Input: part model. Units: mm. Frame: model coordinates. A direction names the side the tool comes from. Coordinates: 2 decimals unless noted, no trailing zeros. Loops run counter-clockwise (first coordinate to the right, second up) from the corner with the lowest first, then second, coordinate; pieces in that order, holes last. Notation, with made-up numbers: M 27.25,50 L 59.25,50 A16 ccw 59.25,76 Z; hole C 69,-11 d11. An arc over 180 degrees is marked long. Use a Markdown table: item, result. Add a question column.
1. Section C-C on y = -2.5. Output: boundary loops of the cut face in (x, z).
2. Section D-D on z = 0. Output: boundary loops of the cut face in (x, y), then the cut area to 3 significant figures.
3. Draft query along X for faces 4 (the flat face through (-5, -0.5, -0.1)), 5 (the flat face through (0, -1, -6)), 6 (the flat face through (0, -4, 10)), 7 (the flat face through (-15.5, -8.5, 0)). Return one class per face: +X half, -X half, draft (parallel to the pull), parting line (faces both ways), or undercut.
4. Section A-A on z = -3. Output: boundary loops of the cut face in (x, y).
5. Pin query (flat end, axial travel): pin 1 (0.5 mm diameter, centred on y = -0.5, z = 1, fed in from +X); pin 2 (1.1 mm diameter, centred on x = 12, y = -8.5, fed in from -Z); pin 3 (2.5 mm diameter, centred on x = 13, z = 0.5, fed in from +Y). Return the tip coordinate at first contact, or that it passes through.
6. Line query: L1, parallel to Z at x = 3.5, y = -4.5; L2, parallel to X at y = -7, z = 4.5; L3, parallel to Z at x = 12, y = -8.35. Output: solid intervals per line, ascending. Write a range as [from, to].
7. Set-up query: faces 1 (the flat face through (-14, -8, 0)), 2 (the flat face through (14, -8, 0)), 3 (the flat face through (5, -0.5, -0.1)). Return all of +Z, -Z, +X, -X, +Y, -Y with unobstructed straight access to the full face (end or side cutting, diameter ignored); none if empty.
8. Section B-B on x = 12. Output: boundary loops of the cut face in (y, z), then the cut area to 3 significant figures.
```python
from build123d import *

# Parameters (mm, degrees)
F0_W     = 21
F0_H     = 20
F0_W_2   = 19
F0_H_2   = 18
F0_W_3   = 18
F0_H_3   = 17
F0_W_4   = 10
F0_H_4   = 10
F1_DEPTH = 1
F2_W     = 21
F2_H     = 20
F2_W_2   = 19
F2_H_2   = 18
F3_DEPTH = 7
F4_W     = 19
F4_H     = 18
F4_W_2   = 5
F4_H_2   = 5
F5_DEPTH = 1
F7_D     = 2


with BuildPart() as f1:
    # F0 (on Front) → F1 (new body)
    with BuildSketch(Plane.XZ):
        Rectangle(F0_W, F0_H)
        Rectangle(F0_W_2, F0_H_2, mode=Mode.SUBTRACT)
        Rectangle(F0_W_2, F0_H_2)
        Rectangle(F0_W_3, F0_H_3, mode=Mode.SUBTRACT)
        Rectangle(F0_W_3, F0_H_3)
        Rectangle(F0_W_4, F0_H_4, mode=Mode.SUBTRACT)
    extrude(amount=F1_DEPTH)

    # F2 (on face) → F3 (join)
    with BuildSketch(Plane.XZ.offset(1)):
        Rectangle(F2_W, F2_H)
        Rectangle(F2_W_2, F2_H_2, mode=Mode.SUBTRACT)
    extrude(amount=F3_DEPTH)

    # F4 (on face) → F5 (join)
    with BuildSketch(Plane.XZ.offset(8)):
        Polygon((10.5, 2.5), (10.5, 10), (-10.5, 10), (-10.5, 2.5), (-10.5, -2.5), (-10.5, -10), (10.5, -10), (10.5, -2.5), align=None)
        Rectangle(F4_W, F4_H, mode=Mode.SUBTRACT)
        with Locations((13, 0)):
            Rectangle(F4_W_2, F4_H_2)
        with Locations((-13, 0)):
            Rectangle(F4_W_2, F4_H_2)
    extrude(amount=F5_DEPTH)

    # F7 (through all)
    with Locations(Plane.XZ.offset(9)):
        with Locations((-12, 0), (12, 0)):
            Hole(F7_D / 2)


solid = f1.part
```
Answers below:
| question | item | result |
|---|---|---|
| 1 | outline | M -10.5,-10 L 10.5,-10 L 10.5,10 L -10.5,10 Z; hole M -9.5,-9 L 9.5,-9 L 9.5,9 L -9.5,9 Z |
| 2 | outline | M -15.5,-9 L -13,-9 L -13,-8 L -15.5,-8 Z; M -11,-9 L -9.5,-9 L -9.5,-1 L -5,-1 L -5,0 L -10.5,0 L -10.5,-8 L -11,-8 Z; M 5,-1 L 9.5,-1 L 9.5,-9 L 11,-9 L 11,-8 L 10.5,-8 L 10.5,0 L 5,0 Z; M 13,-9 L 15.5,-9 L 15.5,-8 L 13,-8 Z |
| 2 | area | 33.0 mm² |
| 3 | face 4 | undercut |
| 3 | face 5 | undercut |
| 3 | face 6 | draft |
| 3 | face 7 | -X half |
| 4 | outline | M -10.5,-9 L -9.5,-9 L -9.5,-1 L -5,-1 L -5,0 L -10.5,0 Z; M 5,-1 L 9.5,-1 L 9.5,-9 L 10.5,-9 L 10.5,0 L 5,0 Z |
| 5 | pin 1 | stops at x = 10.5 |
| 5 | pin 2 | stops at z = -2.5 |
| 5 | pin 3 | stops at y = -8 |
| 6 | L1 | z = [-10, -9], [9, 10] |
| 6 | L2 | x = [-10.5, -9.5], [9.5, 10.5] |
| 6 | L3 | z = [-2.5, -1], [1, 2.5] |
| 7 | face 1 | +Z, -Z, -X, +Y |
| 7 | face 2 | +Z, -Z, +X, +Y |
| 7 | face 3 | +Y, -Y |
| 8 | outline | M -9,-2.5 L -8,-2.5 L -8,-1 L -9,-1 Z; M -9,1 L -8,1 L -8,2.5 L -9,2.5 Z |
| 8 | area | 3.00 mm² |
